Geometry: see drawing. Coordinates: mm, zero at the bounding-box minimum. A direction names the side the tool comes from. Round coordinates to 2 decimals unless told otherwise and drop trailing zeros. Loops run counter-clockwise (first coordinate to the right, second up) from the corner with the lowest first, then second, coordinate; pieces in that order, holes last. Notation, with made-up numbers: (89, -12) -> (116, -12) arc R16 cw to (116, -2) -> close; hole circle Ø2 at (0.25, 7). An arc over 180 degrees is marked (long way). Write item = value, one per line.
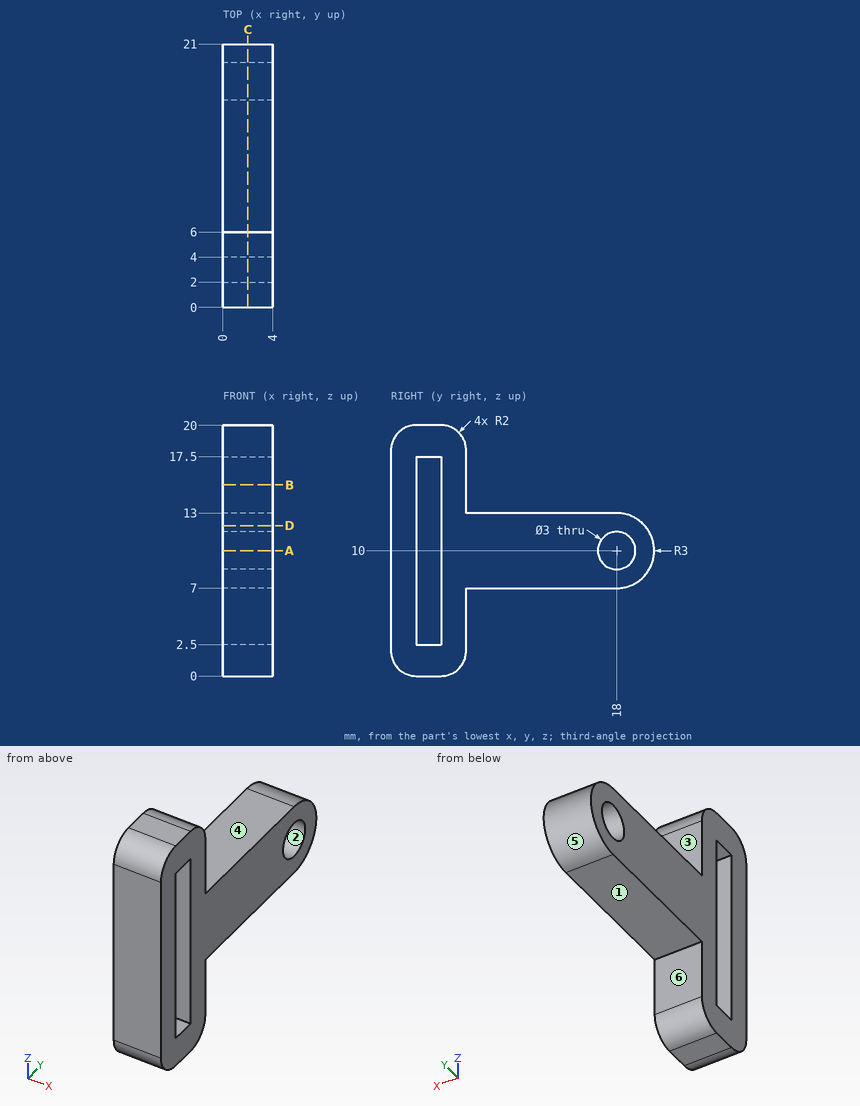
1. Section query A-A (z = 10). Return the cut outline in (x, y).
Evaluation:
outline = (0, 0) -> (4, 0) -> (4, 2) -> (0, 2) -> close; (0, 4) -> (4, 4) -> (4, 16.5) -> (0, 16.5) -> close; (0, 19.5) -> (4, 19.5) -> (4, 21) -> (0, 21) -> close
2. Set-up query: the marked faces 4, 5 and 6. Return all of +Z, -Z, +X, -X, +Y, -Y with unobstructed straight access to the full face (end or side cutting, diameter ignored); none if empty.
Evaluation:
face_4 = +Z, +X, -X, +Y
face_5 = +X, -X, +Y
face_6 = -Z, +X, -X, +Y
3. Section query B-B (z = 15.25). Return the cut outline in (x, y).
Evaluation:
outline = (0, 0) -> (4, 0) -> (4, 2) -> (0, 2) -> close; (0, 4) -> (4, 4) -> (4, 6) -> (0, 6) -> close
4. Section query D-D (z = 12). Return the cut outline in (x, y).
Evaluation:
outline = (0, 0) -> (4, 0) -> (4, 2) -> (0, 2) -> close; (0, 4) -> (4, 4) -> (4, 20.24) -> (0, 20.24) -> close
5. Mould query, pull axis Y, two halves, no side actions, for the marked faces 1, 2 and 3. Classes: released by +Y, released by -Y, zero draft, split by the parting line, or undercut.
Evaluation:
face_1 = zero draft
face_2 = undercut
face_3 = released by +Y
6. Line query: probe 1 along Y at (x, z) = (1.05, 10); probe 2 along Y at (x, z) = (1.6, 5.5); probe 3 along Z at (x, y) = (3.85, 3). Output: solid intervals per line, ascending. Write a range as from..to.
Evaluation:
probe_1 = 0..2, 4..16.5, 19.5..21
probe_2 = 0..2, 4..6
probe_3 = 0..2.5, 17.5..20
7. Contact query for flat-ended pins moving along their axis: pin 1 Ø1.5 at (y, z) = (14.5, 4.5) entering from -X; pin 2 Ø1.5 at (x, z) = (2, 14.5) entering from -Y; pin 3 Ø2 at (x, y) = (1, 14.5) entering from +Z; pin 4 Ø1.2 at (x, y) = (2.5, 10.5) entering from -Z. Output: stop coordinate, or through.
Evaluation:
pin_1 = through
pin_2 = 0
pin_3 = 13
pin_4 = 7
8. Section query C-C (x = 2). Return the cut outline in (y, z), then the cut area to 3 significant figures.
Evaluation:
outline = (0, 2) arc R2 ccw to (2, 0) -> (4, 0) arc R2 ccw to (6, 2) -> (6, 7) -> (18, 7) arc R3 ccw to (18, 13) -> (6, 13) -> (6, 18) arc R2 ccw to (4, 20) -> (2, 20) arc R2 ccw to (0, 18) -> close; hole (2, 2.5) -> (4, 2.5) -> (4, 17.5) -> (2, 17.5) -> close; hole circle Ø3 at (18, 10)
area = 166 mm²
